Work out the finished part from the listing and answer in its coordinate system (mm). A direction names the side the tool comes from. Give positions to 0.01 mm unless a question says otherwise; leave off trailing zeros. Write each loop counter-clockwise with the first axis right and the second up, starting at its lowest first coordinate (ties: lowest second). Pieces come first, ordered by that corner, then holes. Notation, with made-up numbers: (27.5, 23) -> (72.5, 23) arc R29 cw to (72.5, 53) -> close; hole circle Ø10 at (31, 1). An arc over 180 degrees is marked (long way). Write item = value, one per line. Start each with the question number.
from build123d import *

# Parameters (mm, degrees)
F0_R     = 1.2
F1_DEPTH = 1
F2_DEPTH = 7.4
F3_DEPTH = 5


with BuildPart() as f1:
    # F0 (on Top) → F1 (new body)
    with BuildSketch(Plane.XY):
        Polygon((34.807068, -8.220604), (15.057068, -8.220604), (15.057068, -18.220604), (16.057068, -18.220604), (16.057068, -19.220604), (33.807068, -19.220604), (33.807068, -18.220604), (34.807068, -18.220604), align=None)
        with Locations((20.057068, -16.020604)):
            Circle(F0_R, mode=Mode.SUBTRACT)
        with Locations((29.557068, -16.020604)):
            Circle(F0_R, mode=Mode.SUBTRACT)
    extrude(amount=F1_DEPTH)

    # F0 (on Top) → F2 (join)
    with BuildSketch(Plane.XY):
        Polygon((15.057068, -8.220604), (13.057068, -8.220604), (13.057068, -19.220604), (16.057068, -19.220604), (16.057068, -18.220604), (15.057068, -18.220604), align=None)
        Polygon((36.807068, -8.220604), (34.807068, -8.220604), (34.807068, -18.220604), (33.807068, -18.220604), (33.807068, -19.220604), (36.807068, -19.220604), align=None)
    extrude(amount=F2_DEPTH)

    # F0 (on Top) → F3 (join)
    with BuildSketch(Plane.XY):
        with Locations((20.057068, -16.020604)):
            Circle(F0_R)
        with Locations((29.557068, -16.020604)):
            Circle(F0_R)
    extrude(amount=F3_DEPTH)


solid = f1.part
(1) Each of these flat-tipped pins is pushed along its axis until it touches: pin 1 (1.1 mm diameter, centred on x = 16, z = 4.5, fed in from +Y); pin 2 (1.2 mm diameter, centred on x = 29, y = -16, fed in from +Z); pin 3 (1.5 mm diameter, centred on x = 22.5, z = 5, fed in from -Y); pin 4 (3.5 mm diameter, centred on x = 28, y = -12, fed in from +Z). Where does it stop, or does it pass through?
(2) Determine the mould class of faces 6 (the flat face through (36.807, -14, 4)), 7 (the flat face through (15.6, -18.221, 4.2)), 8 (the flat face through (14, -14, 7.4)) for opening direction X: pulls with the +X half, pulls with the -X half, needs draft (parallel to the pull), parting line crosses it, or undercut.
(3) Find the intervals of material crossed by line 1 along X through (y, z) = (-16.5, 6.5); line 2 along X through (y, z) = (-15.5, 3); line 3 along Z through (x, y) = (22.5, -13.25), in increasing order.
(4) A cutting plane is placed at B-B, the plane y = -14. Write down the section's boundary in (x, z).
(5) A cutting plane is placed at C-C, the plane x = 29.75. Write down the section's boundary in (y, z) (3 decimals).
(6) For faces 1 (the flat face through (13.057, -14, 4)), 2 (the flat face through (34.807, -13, 4)), 3 (the cylindrical face through (21.2, -15.66, 2.97)), 4 (the flat face through (25, -14, 0)), 5 (the flat face through (20, -16, 5)), determine the directions among +Z, -Z, +X, -X, +Y, -Y from which every point of the face is accessible in a straight line to the end or side of a thin tool.
(7) A cutting plane is placed at A-A, the plane z = 5.5. Write down the section's boundary in (x, y).
(8) A cutting plane is placed at D-D, the plane z = 3.75. Write down the section's boundary in (x, y).
Results list:
q1.pin_1 = -18.22
q1.pin_2 = 5
q1.pin_3 = through
q1.pin_4 = 1
q2.face_6 = pulls with the +X half
q2.face_7 = undercut
q2.face_8 = needs draft
q3.line_1 = 13.06 to 15.06, 34.81 to 36.81
q3.line_2 = 13.06 to 15.06, 18.98 to 21.14, 28.48 to 30.64, 34.81 to 36.81
q3.line_3 = 0 to 1
q4.outline = (13.06, 0) -> (36.81, 0) -> (36.81, 7.4) -> (34.81, 7.4) -> (34.81, 1) -> (15.06, 1) -> (15.06, 7.4) -> (13.06, 7.4) -> close
q5.outline = (-19.221, 0) -> (-8.221, 0) -> (-8.221, 1) -> (-14.836, 1) -> (-14.836, 5) -> (-17.205, 5) -> (-17.205, 1) -> (-19.221, 1) -> close
q6.face_1 = +Z, -Z, -X, +Y, -Y
q6.face_2 = +Z, +Y
q6.face_3 = +Z
q6.face_4 = -Z, +X, -X, +Y, -Y
q6.face_5 = +Z, +Y, -Y
q7.outline = (13.06, -19.22) -> (16.06, -19.22) -> (16.06, -18.22) -> (15.06, -18.22) -> (15.06, -8.22) -> (13.06, -8.22) -> close; (33.81, -19.22) -> (36.81, -19.22) -> (36.81, -8.22) -> (34.81, -8.22) -> (34.81, -18.22) -> (33.81, -18.22) -> close
q8.outline = (13.06, -19.22) -> (16.06, -19.22) -> (16.06, -18.22) -> (15.06, -18.22) -> (15.06, -8.22) -> (13.06, -8.22) -> close; circle Ø2.4 at (20.06, -16.02); circle Ø2.4 at (29.56, -16.02); (33.81, -19.22) -> (36.81, -19.22) -> (36.81, -8.22) -> (34.81, -8.22) -> (34.81, -18.22) -> (33.81, -18.22) -> close
